Verification items for the finished model (mm, model axes). A direction names the side the tool comes from. Round coordinates to 2 decimals unless told otherwise and drop trailing zeros. Write each loop counter-clockwise with the first axis right and the second up, starting at its lowest first coordinate (ties: lowest second). Pieces come first, ordered by that corner, then holes. Notation, with made-up numbers: M 24.25,19.5 L 61.25,19.5 A14 cw 61.25,23.5 Z; hole C 33.5,-25.75 d8. An arc over 180 degrees is marked long. Use a Markdown table: item, result. Add a question column.
from build123d import *

# Parameters (mm, degrees)
F0_W     = 19.6
F0_H     = 19.6
F1_DEPTH = 21.5
F2_W     = 17.6
F2_H     = 17.6
F3_DEPTH = 10.5
F4_W     = 17.6
F4_H     = 17.6
F5_DEPTH = 10
F6_R     = 1.75
F7_DEPTH = 1


with BuildPart() as f1:
    # F0 (on Top) → F1 (new body)
    with BuildSketch(Plane.XY):
        Rectangle(F0_W, F0_H)
    extrude(amount=F1_DEPTH)

    # F2 (on face) → F3 (cut)
    with BuildSketch(Plane(origin=(0, 0, 0), x_dir=(1, 0, 0), z_dir=(0, 0, -1))):
        Rectangle(F2_W, F2_H)
    extrude(amount=-F3_DEPTH, mode=Mode.SUBTRACT)

    # F4 (on face) → F5 (cut)
    with BuildSketch(Plane.XY.offset(21.5)):
        Rectangle(F4_W, F4_H)
    extrude(amount=-F5_DEPTH, mode=Mode.SUBTRACT)

    # F6 (on face) → F7 (cut)
    with BuildSketch(Plane.XY.offset(11.5)):
        Circle(F6_R)
    extrude(amount=-F7_DEPTH, mode=Mode.SUBTRACT)


solid = f1.part
1. Access from +Z, -Z, +X, -X, +Y, -Y to the whole of each face (thin tool, end or side, straight path). Record for faces 5 (the flat face through (-8.8, 0, 5)), 6 (the flat face through (0, -8.8, 17)), 7 (the cylindrical face through (1.617, -0.67, 11.007)).
2. Depth check by flat-ended pin: pin 1 Ø2 at (x, y) = (0, 0) entering from -Z; pin 2 Ø2 at (x, y) = (-7, -2.5) entering from -Z; pin 3 Ø9 at (x, y) = (4, 0) entering from +Z. Enter the tip coordinate at first touch or a pass-through.
3. Release check for a two-part mould opening along X. For faces 1 (the flat face through (-9.8, 0, 11)), 2 (the flat face through (9.8, 0, 11)), 3 (the flat face through (-2, 0, 11.5)), 4 (the flat face through (0, 9.8, 11)) record: +X half, -X half, draft (parallel to the pull), parting line (faces both ways), or undercut.
4. Cross-section at D-D on x = 7.5. Enter the section's corners in (y, z).
5. Scan lines: line 1 along X through (y, z) = (-2.75, 4.75); line 2 along Y through (x, z) = (0, 11.15). Record each from-to range of solid material in increasing order. Write a range as from..to.
6. Cross-section at A-A on y = 0. Enter the section's corners in (x, z), plus the area to 3 significant figures.
7. Cross-section at B-B on z = 17.75. Enter the section's corners in (x, y), plus the area to 3 significant figures.
Answer:
| question | item | result |
|---|---|---|
| 1 | face 5 | -Z |
| 1 | face 6 | +Z |
| 1 | face 7 | +Z, -Z |
| 2 | pin 1 | passes through |
| 2 | pin 2 | stops at z = 10.5 |
| 2 | pin 3 | stops at z = 11.5 |
| 3 | face 1 | -X half |
| 3 | face 2 | +X half |
| 3 | face 3 | undercut |
| 3 | face 4 | draft |
| 4 | outline | M -9.8,0 L -8.8,0 L -8.8,10.5 L 8.8,10.5 L 8.8,0 L 9.8,0 L 9.8,21.5 L 8.8,21.5 L 8.8,11.5 L -8.8,11.5 L -8.8,21.5 L -9.8,21.5 Z |
| 5 | line 1 | x = -9.8..-8.8, 8.8..9.8 |
| 5 | line 2 | y = -9.8..-1.75, 1.75..9.8 |
| 6 | outline | M -9.8,0 L -8.8,0 L -8.8,10.5 L -1.75,10.5 L -1.75,11.5 L -8.8,11.5 L -8.8,21.5 L -9.8,21.5 Z; M 1.75,10.5 L 8.8,10.5 L 8.8,0 L 9.8,0 L 9.8,21.5 L 8.8,21.5 L 8.8,11.5 L 1.75,11.5 Z |
| 6 | area | 57.1 mm^2 |
| 7 | outline | M -9.8,-9.8 L 9.8,-9.8 L 9.8,9.8 L -9.8,9.8 Z; hole M -8.8,-8.8 L 8.8,-8.8 L 8.8,8.8 L -8.8,8.8 Z |
| 7 | area | 74.4 mm^2 |
